Design review of the part built by this model. Coordinates are the model's own, in mm. Coordinates: 2 decimals unless noted, no trailing zeros. Loops run counter-clockwise (first coordinate to the right, second up) from the corner with the lowest first, then second, coordinate; pieces in that order, holes last. Notation, with made-up numbers: (27, -39) -> (85, -39) arc R17 cw to (85, -27) -> close; hole circle Ø1 at (48, -11). An arc over 180 degrees is marked (long way). Use a Markdown table: item, result. Add a question column.
Q1. Take a section at B-B on x = 41.5. Write out the cut boundary in (y, z).
Q2. Take a section at D-D on y = 0.95. Count the separate pieces of the cut face and the enclosed holes in it, plus the area to 3 significant figures.
Q3. For probe 1 along X at (y, z) = (2.3, 6); probe 2 along Z at (x, y) = (48, 1.8); probe 3 along X at (y, z) = (1.6, -36.5), list the stretches that pass through material, from the lowest coordinate up.
Q4. Clearance check with flat-ended pins moving along their axes: pin 1 Ø1.5 at (y, z) = (1, -31) entering from -X; pin 2 Ø0.9 at (y, z) = (2, -18.5) entering from -X; pin 3 Ø9 at (x, z) = (38.41, -49.5) entering from -Y; pin 4 Ø0.9 at (x, y) = (46.5, 2) entering from +Z. State where each tip first meets the part, or that it passes through.
Q5. Take a section at C-C on z = 1. Write out the cut boundary in (x, y).
Q6. Take a section at A-A on z = -67. Write out the cut boundary in (x, y), plus the area to 3 significant figures.
from build123d import *

# Parameters (mm, degrees)
SKETCH1_R           = 5
SKETCH1_R_2         = 1.5
BOSS_EXTRUDE1_DEPTH = 3
FILLET1_R           = 3
SKETCH2_W           = 8
SKETCH2_H           = 49
CUT_EXTRUDE1_DEPTH  = 104.979147454
FILLET2_R           = 2


with BuildPart() as part:
    # Sketch1 → Boss-Extrude1 (new body)
    with BuildSketch(Plane(origin=(0, 0, 0), x_dir=(1, 0, 0), z_dir=(0, 1, 0))):
        with BuildLine():
            Line((10.905619524, 39.769696007), (10.905619524, 61))
            Line((10.905619524, 61), (10.905619524, 71))
            Line((10.905619524, 71), (18.905619524, 71))
            Line((18.905619524, 71), (18.905619524, 61))
            Line((18.905619524, 61), (67.905619524, 61))
            Line((67.905619524, 61), (67.905619524, 71))
            Line((67.905619524, 71), (75.905619524, 71))
            Line((75.905619524, 71), (75.905619524, 61))
            Line((75.905619524, 61), (75.905619524, 0))
            Line((75.905619524, 0), (75.905619524, -10))
            Line((75.905619524, -10), (67.905619524, -10))
            Line((67.905619524, -10), (67.905619524, 0))
            Line((67.905619524, 0), (18.905619524, 0))
            Line((18.905619524, 0), (18.905619524, -10))
            Line((18.905619524, -10), (10.905619524, -10))
            Line((10.905619524, -10), (10.905619524, 0))
            Line((10.905619524, 0), (10.905619524, 20.230303993))
            ThreePointArc((10.905619524, 20.230303993), (17.347708153, 24.241211504), (12.405619524, 30))
            ThreePointArc((12.405619524, 30), (17.347708153, 35.758788496), (10.905619524, 39.769696007))
        make_face()
        with Locations(Location((38.405619524, 10.5, 0), (0, 0, 270))):
            Circle(SKETCH1_R, mode=Mode.SUBTRACT)
        with Locations(Location((38.405619524, 49.5, 0), (0, 0, 270))):
            Circle(SKETCH1_R, mode=Mode.SUBTRACT)
        with Locations(Location((14.905619524, -6, 0), (0, 0, 270))):
            Circle(SKETCH1_R_2, mode=Mode.SUBTRACT)
        with Locations(Location((14.905619524, 67, 0), (0, 0, 90))):
            Circle(SKETCH1_R_2, mode=Mode.SUBTRACT)
        with Locations(Location((71.905619524, -6, 0), (0, 0, 270))):
            Circle(SKETCH1_R_2, mode=Mode.SUBTRACT)
        with Locations(Location((71.905619524, 67, 0), (0, 0, 90))):
            Circle(SKETCH1_R_2, mode=Mode.SUBTRACT)
    extrude(amount=BOSS_EXTRUDE1_DEPTH)

    # Fillet1
    fillet1_edges = [part.edges().sort_by_distance(p)[0] for p in [
        (10.905619524, 1.5, -20.230303993),
        (12.405619524, 1.5, -30),
        (10.905619524, 1.5, -39.769696007),
        (10.905619524, 1.5, -71),
        (18.905619524, 1.5, -71),
        (18.905619524, 1.5, -61),
        (67.905619524, 1.5, -61),
        (67.905619524, 1.5, -71),
        (75.905619524, 1.5, -71),
        (75.905619524, 1.5, 10),
        (67.905619524, 1.5, 10),
        (67.905619524, 1.5, 0),
        (18.905619524, 1.5, 0),
        (18.905619524, 1.5, 10),
        (10.905619524, 1.5, 10),
    ]]
    fillet(fillet1_edges, radius=FILLET1_R)

    # Sketch2 → Cut-Extrude1 (cut, through all)
    with BuildSketch(Plane(origin=(0, 3, 0), x_dir=(1, 0, 0), z_dir=(0, 1, 0))):
        Polygon((53.314584868, 30.5), (30.951136852, 43.411542732), (30.951136852, 17.588457268), align=None)
        Polygon((69.905619524, 27.5), (69.905619524, 1.676914536), (47.542171508, 14.588457268), align=None)
        Polygon((47.542171508, 46.411542732), (69.905619524, 33.5), (69.905619524, 59.323085464), align=None)
        Polygon((69.654975177, 30.5), (46.180472316, 44.053010546), (43.457073931, 39.335946174), (58.761381637, 30.5), (43.457073931, 21.664053826), (46.180472316, 16.946989454), align=None)
        with Locations((23.951136852, 30)):
            Rectangle(SKETCH2_W, SKETCH2_H)
    extrude(amount=-CUT_EXTRUDE1_DEPTH, mode=Mode.SUBTRACT)

    # Fillet2
    fillet2_edges = [part.edges().sort_by_distance(p)[0] for p in [
        (53.314584868, 1.5, -30.5),
        (30.951136852, 1.5, -17.588457268),
        (30.951136852, 1.5, -43.411542732),
        (47.542171508, 1.5, -14.588457268),
        (69.905619524, 1.5, -27.5),
        (69.905619524, 1.5, -1.676914536),
        (47.542171508, 1.5, -46.411542732),
        (69.905619524, 1.5, -59.323085464),
        (69.905619524, 1.5, -33.5),
        (43.457073931, 1.5, -39.335946174),
        (46.180472316, 1.5, -44.053010546),
        (69.654975177, 1.5, -30.5),
        (46.180472316, 1.5, -16.946989454),
        (43.457073931, 1.5, -21.664053826),
        (58.761381637, 1.5, -30.5),
        (27.951136852, 1.5, -54.5),
        (27.951136852, 1.5, -5.5),
        (19.951136852, 1.5, -5.5),
        (19.951136852, 1.5, -54.5),
    ]]
    fillet(fillet2_edges, radius=FILLET2_R)


solid = part.part
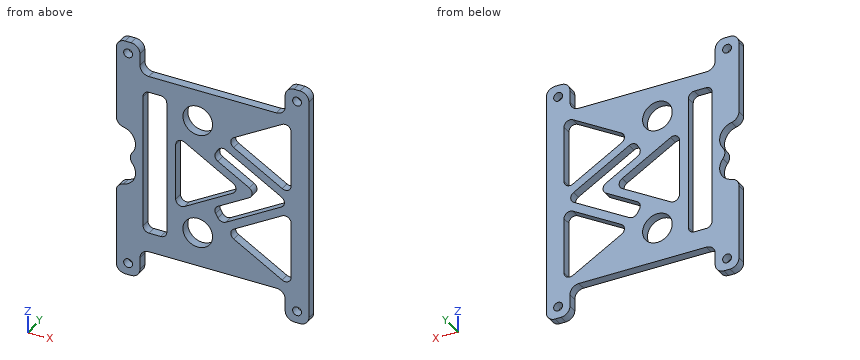
Answer list:
| question | item | result |
|---|---|---|
| 1 | outline | (0, -61) -> (3, -61) -> (3, -53.43) -> (0, -53.43) -> close; (0, -45.57) -> (3, -45.57) -> (3, -37.32) -> (0, -37.32) -> close; (0, -23.68) -> (3, -23.68) -> (3, -14.43) -> (0, -14.43) -> close; (0, -6.57) -> (3, -6.57) -> (3, 0) -> (0, 0) -> close |
| 2 | separate pieces | 1 |
| 2 | enclosed holes | 11 |
| 2 | area | 2,510 mm² |
| 3 | probe 1 | 10.91 to 13.41, 16.41 to 18.91, 67.91 to 70.41, 73.41 to 75.91 |
| 3 | probe 2 | -61 to -43, -36.71 to -33.57, -27.43 to -24.29, -18 to 0 |
| 3 | probe 3 | 17.18 to 19.95, 27.95 to 30.95, 42.92 to 48.37, 59.26 to 64.71, 69.85 to 75.91 |
| 4 | pin 1 | x = 15.66 |
| 4 | pin 2 | x = 11.05 |
| 4 | pin 3 | through |
| 4 | pin 4 | z = 0 |
| 5 | outline | (10.91, 0) -> (19.67, 0) -> (19.67, 3) -> (10.91, 3) -> close; (67.14, 0) -> (75.91, 0) -> (75.91, 3) -> (67.14, 3) -> close |
| 6 | outline | (10.91, 0) -> (13.41, 0) -> (13.41, 3) -> (10.91, 3) -> close; (16.41, 0) -> (18.91, 0) -> (18.91, 3) -> (16.41, 3) -> close; (67.91, 0) -> (70.41, 0) -> (70.41, 3) -> (67.91, 3) -> close; (73.41, 0) -> (75.91, 0) -> (75.91, 3) -> (73.41, 3) -> close |
| 6 | area | 30.0 mm² |
